The model under review builds one solid part; all positions refer to its coordinate system, in mm. Face numbers are marked on the shaded views. A direction names the side the tool comes from. Give positions to 0.01 mm unless a question says otherwise; leave off trailing zeros. Order: outer loops, then holes, each group sorted by start corner. A loop starts at its lowest first (then second) coordinate and runs counter-clockwise, first axis right, second up. Notation, with made-up numbers: M 45.5,71.25 L 51.5,71.25 A17 cw 51.5,96.25 Z; hole C 23,-24.75 d7. An arc over 180 degrees is marked long. One line per question, with ' | ' between items. Start each with the question number.
1. The part is to be moulded in two halves that separate along Y. For the marked faces 1 and 2, say which applies: +Y half, -Y half, draft (parallel to the pull), parting line (faces both ways), or undercut.
2. We need section A-A on x = -1.75. Write out the cut boundary in (y, z).
3. We need section D-D on x = 18.5. Write out the cut boundary in (y, z).
4. We need section C-C on z = 0.25. Count the separate pieces of the cut face and the enclosed holes in it, then the cut area to 3 significant figures.
5. For the marked faces 3, 4, 5 and 6, list the 3-axis set-ups (+Z, -Z, +X, -X, +Y, -Y) from which the entire face can be reached by the end or side of a thin tool; tool diameter is ignored.
6. We need section B-B on y = 13.5. Write out the cut boundary in (x, z), then the cut area to 3 significant figures.
7. Wall thickness on L1, parallel to X at y = 1.75, z = 0.95; L2, parallel to X at y = 14, z = 0.2; L3, parallel to Y at x = 21, z = 1.4: over which ranges is each line inside the solid? List them lowest first.
8. Insertion check: P1, Ø0.8, axis at y = 3.5, z = 0.5, coming from the -X side; P2, Ø0.5, axis at x = -4.5, z = 1, coming from the -Y side; P3, Ø0.5, axis at x = -4, z = 0.5, coming from the +Y side; P4, Ø2.5, axis at x = 23.495, y = 8.255, coming from the +Z side. Each pin has a flat end and moves straight along its axis. Give the tip position at first contact, or say it passes through.
```python
from build123d import *

# Parameters (mm, degrees)
BOARD_OUTLINE_DEPTH = 1.6
SKETCH2_R           = 0.3
SKETCH2_R_2         = 0.127
SKETCH2_R_3         = 0.1651
SKETCH2_R_4         = 0.2032
SKETCH2_R_5         = 1.5
NPTH_DEPTH          = 2.6
SKETCH3_R           = 1.27
PTH_DEPTH           = 2.6


with BuildPart() as part:
    # Sketch1 → Board_Outline (new body)
    with BuildSketch(Plane.XY):
        Polygon((0, 16.51), (0, 11.176), (-6.731, 11.176), (-7.468412, 11.062199), (-8.151243, 10.761418), (-8.732959, 10.294157), (-9.173918, 9.692258), (-9.444069, 8.996739), (-9.525, 8.255), (-9.444069, 7.513261), (-9.173918, 6.817742), (-8.732959, 6.215843), (-8.151243, 5.748582), (-7.468412, 5.447801), (-6.731, 5.334), (0, 5.334), (0, 0), (16.51, 0), (16.51, 5.334), (23.241, 5.334), (23.978412, 5.447801), (24.661243, 5.748582), (25.242959, 6.215843), (25.683918, 6.817742), (25.954069, 7.513261), (26.035, 8.255), (25.954069, 8.996739), (25.683918, 9.692258), (25.242959, 10.294157), (24.661243, 10.761418), (23.978412, 11.062199), (23.241, 11.176), (16.51, 11.176), (16.51, 16.51), align=None)
    extrude(amount=BOARD_OUTLINE_DEPTH)

    # Sketch2 → NPTH (cut, through all)
    with BuildSketch(Plane.XY):
        with Locations((13.555, 14.2)):
            Circle(SKETCH2_R)
        with Locations((2.955, 14.2)):
            Circle(SKETCH2_R)
        with Locations((9.1948, 7.8994)):
            Circle(SKETCH2_R_2)
        with Locations((10.4648, 5.4864)):
            Circle(SKETCH2_R_2)
        with Locations((11.2268, 5.4864)):
            Circle(SKETCH2_R_2)
        with Locations((10.4648, 6.1214)):
            Circle(SKETCH2_R_2)
        with Locations((10.414, 15.7988)):
            Circle(SKETCH2_R_2)
        with Locations((5.005, 9.727)):
            Circle(SKETCH2_R_2)
        with Locations((6.8072, 8.636)):
            Circle(SKETCH2_R_2)
        with Locations((4.699, 8.382)):
            Circle(SKETCH2_R_2)
        with Locations((10.922, 8.636)):
            Circle(SKETCH2_R_2)
        with Locations((6.378, 16.129)):
            Circle(SKETCH2_R_2)
        with Locations((6.8072, 7.874)):
            Circle(SKETCH2_R_2)
        with Locations((6.878, 15.748)):
            Circle(SKETCH2_R_2)
        with Locations((7.378, 16.141)):
            Circle(SKETCH2_R_2)
        with Locations((7.5946, 7.1186)):
            Circle(SKETCH2_R_2)
        with Locations((8.509, 15.748)):
            Circle(SKETCH2_R_2)
        with Locations((5.588, 7.239)):
            Circle(SKETCH2_R_2)
        with Locations((9.779, 15.748)):
            Circle(SKETCH2_R_2)
        with Locations((9.906, 8.636)):
            Circle(SKETCH2_R_2)
        with Locations((9.194, 7.112)):
            Circle(SKETCH2_R_2)
        with Locations((9.144, 15.748)):
            Circle(SKETCH2_R_2)
        with Locations((5.588, 7.874)):
            Circle(SKETCH2_R_2)
        with Locations((13.335, 6.096)):
            Circle(SKETCH2_R_3)
        with Locations((12.319, 1.778)):
            Circle(SKETCH2_R_4)
        with Locations((13.716, 8.509)):
            Circle(SKETCH2_R_4)
        with Locations((2.286, 6.731)):
            Circle(SKETCH2_R_4)
        with Locations((6.985, 4.445)):
            Circle(SKETCH2_R_3)
        with Locations((3.048, 4.445)):
            Circle(SKETCH2_R_3)
        with Locations((11.505, 9.45)):
            Circle(SKETCH2_R_2)
        with Locations((8.386, 9.267)):
            Circle(SKETCH2_R_2)
        with Locations((4.826, 15.748)):
            Circle(SKETCH2_R_2)
        with Locations((4.191, 15.748)):
            Circle(SKETCH2_R_2)
        with Locations((-6.985, 8.255)):
            Circle(SKETCH2_R_5)
        with Locations((23.495, 8.255)):
            Circle(SKETCH2_R_5)
        with Locations((13.716, 11.176)):
            Circle(SKETCH2_R_4)
        with Locations((2.286, 10.541)):
            Circle(SKETCH2_R_4)
        with Locations((14.478, 15.113)):
            Circle(SKETCH2_R_3)
        with Locations((13.462, 15.113)):
            Circle(SKETCH2_R_3)
        with Locations((14.478, 14.224)):
            Circle(SKETCH2_R_3)
        with Locations((5.505, 15.748)):
            Circle(SKETCH2_R_2)
        with Locations((3.429, 14.859)):
            Circle(SKETCH2_R_2)
        with Locations((7.874, 15.748)):
            Circle(SKETCH2_R_2)
        with Locations((11.5062, 15.748)):
            Circle(SKETCH2_R_2)
        with Locations((13.462, 1.778)):
            Circle(SKETCH2_R_4)
        with Locations((14.732, 1.778)):
            Circle(SKETCH2_R_4)
        with Locations((15.367, 16.002)):
            Circle(SKETCH2_R_4)
    extrude(amount=NPTH_DEPTH, mode=Mode.SUBTRACT)

    # Sketch3 → PTH (cut, through all)
    with BuildSketch(Plane.XY):
        with Locations((-1.75, 8.26)):
            Circle(SKETCH3_R)
        with Locations((18.26, 8.26)):
            Circle(SKETCH3_R)
    extrude(amount=PTH_DEPTH, mode=Mode.SUBTRACT)


solid = part.part
```
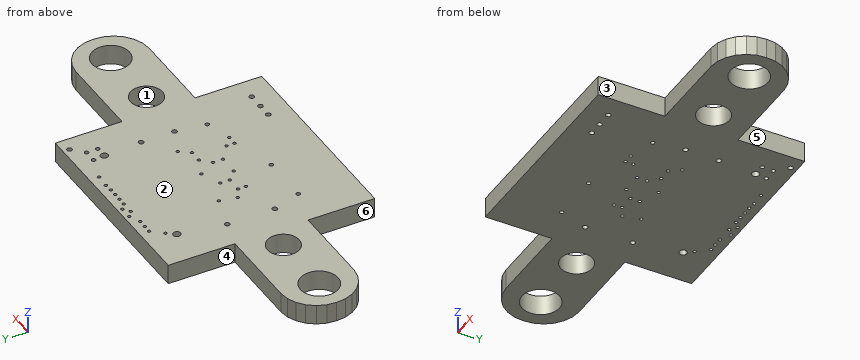
Entries:
1) face 1: undercut | face 2: draft
2) outline: M 5.33,0 L 6.99,0 L 6.99,1.6 L 5.33,1.6 Z; M 9.53,0 L 11.18,0 L 11.18,1.6 L 9.53,1.6 Z
3) outline: M 5.33,0 L 7.01,0 L 7.01,1.6 L 5.33,1.6 Z; M 9.51,0 L 11.18,0 L 11.18,1.6 L 9.51,1.6 Z
4) separate pieces: 1 | enclosed holes: 49 | area: 349 mm^2
5) face 3: +Z, -Z, +X, -Y | face 4: +Z, -Z, -X, +Y | face 5: +Z, -Z, +X, +Y | face 6: +Z, -Z, -X, -Y
6) outline: M 0,0 L 16.51,0 L 16.51,1.6 L 0,1.6 Z | area: 26.4 mm^2
7) L1: x = 0 to 12.12, 12.52 to 13.26, 13.66 to 14.53, 14.93 to 16.51 | L2: x = 0 to 2.73, 3.18 to 13.33, 13.78 to 16.51 | L3: y = 5.33 to 11.18
8) P1: stops at x = 0 | P2: stops at y = 5.33 | P3: stops at y = 11.18 | P4: passes through
